Answer from the drawing. Dimensions are ordinates in mm from the lowest x, y and z of the part. A direction names the side the tool comes from. Coordinates: 2 decimals unless noted, no trailing zeros. Order: outer loops, then holes, each group sorted by start corner. A loop starts at its lowest first (then second) coordinate and runs counter-clockwise, first axis right, second up.
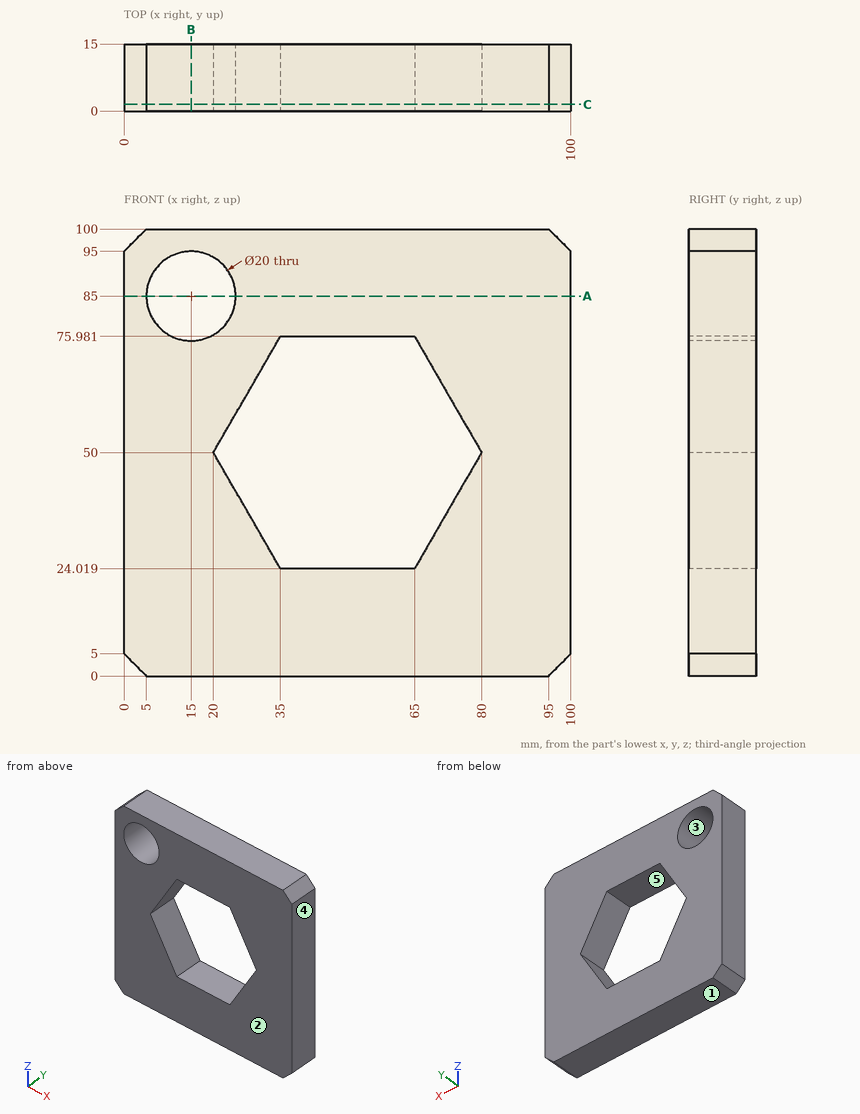
1. The part is cut by section B-B (x = 15). Determine the outline of the cut face in (y, z), plus the area to 3 significant figures.
2. Consider probe 1 along Z at (x, y) = (58, 2); probe 2 along Z at (x, y) = (15, 11.5); probe 3 along X at (y, z) = (12.75, 38). Determine where each line is inside the solid, lowest interval first.
3. The part is cut by section C-C (y = 1.5). Determine the outline of the cut face in (x, z), plus the area to 3 significant figures.
4. The mould has two halves that part along Z. Classify the marked faces 1, 2 and 3: released by +Z, released by -Z, zero draft, split by the parting line, or undercut.
5. The part is cut by section A-A (z = 85). Determine the outline of the cut face in (x, y).
6. For the marked faces 4 and 5, determine the directions among +Z, -Z, +X, -X, +Y, -Y from which every point of the face is accessible in a straight line to the end or side of a thin tool.
Worked out:
1. outline: (0, 0) - (15, 0) - (15, 75) - (0, 75) - close; (0, 95) - (15, 95) - (15, 100) - (0, 100) - close
1. area: 1,200 mm2
2. probe 1: z = 0 to 24.02, 75.98 to 100
2. probe 2: z = 0 to 75, 95 to 100
2. probe 3: x = 0 to 26.93, 73.07 to 100
3. outline: (0, 5) - (5, 0) - (95, 0) - (100, 5) - (100, 95) - (95, 100) - (5, 100) - (0, 95) - close; hole circle Ø20 at (15, 85); hole (20, 50) - (35, 24.02) - (65, 24.02) - (80, 50) - (65, 75.98) - (35, 75.98) - close
3. area: 7,300 mm2
4. face 1: released by -Z
4. face 2: zero draft
4. face 3: undercut
5. outline: (0, 0) - (5, 0) - (5, 15) - (0, 15) - close; (25, 0) - (100, 0) - (100, 15) - (25, 15) - close
6. face 4: +Z, -Z, +X, +Y, -Y
6. face 5: +Y, -Y
